Geometry check sheet. Reference: drawing and pictorial views, mm from the part's lowest x, y, z. Give positions to 0.01 mm unless a question says otherwise; leave off trailing zeros. Order: outer loops, then holes, each group sorted by start corner. A loop starts at its lowest first (then second) coordinate and runs counter-clockwise, first axis right, second up.
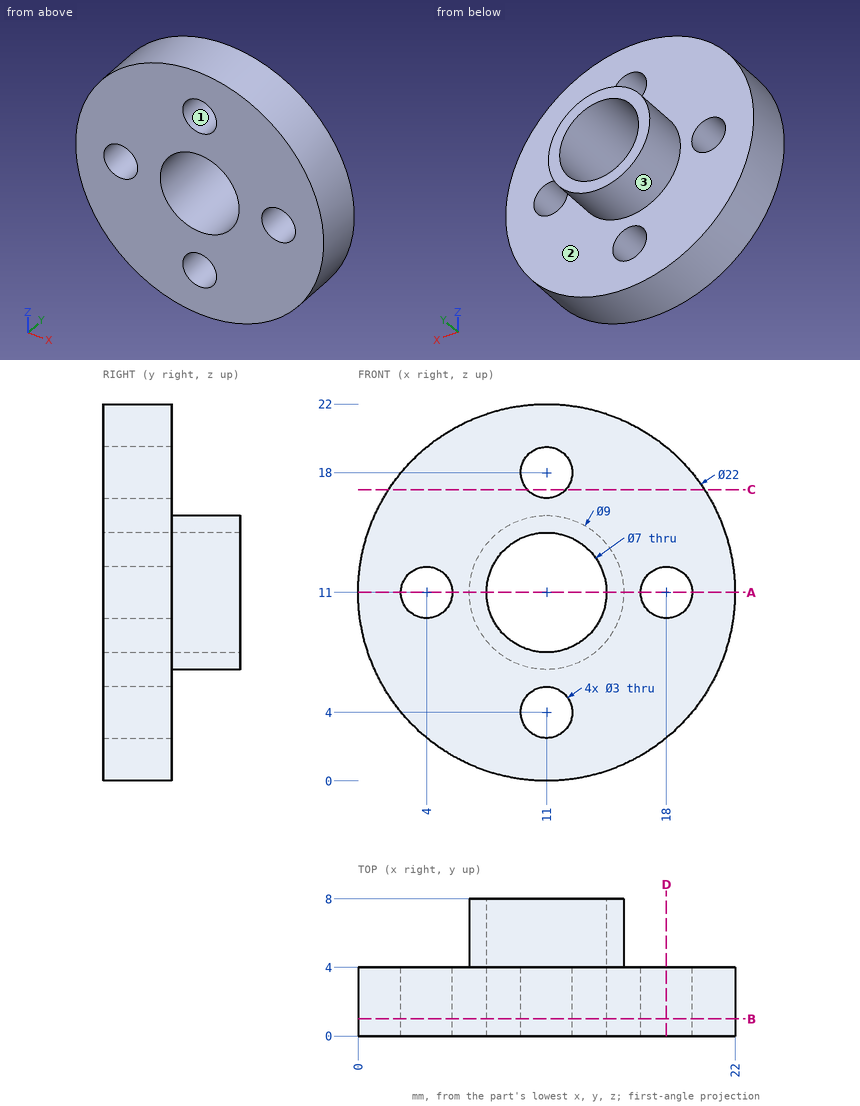
(1) Material ranges on L1, parallel to X at y = 0.9, z = 11; L2, parallel to Z at x = 10, y = 1.25; L3, parallel to Y at x = 5.75, z = 13.5, recorded low to high.
Response values:
L1: x = 0 to 2.5, 5.5 to 7.5, 14.5 to 16.5, 19.5 to 22
L2: z = 0.05 to 2.88, 5.12 to 7.65, 14.35 to 16.88, 19.12 to 21.95
L3: y = 0 to 4
(2) Cross-section at C-C on z = 17. Enter the section's corners in (x, y), then the cut area to 3 significant figures.
Response values:
outline: (1.78, 0) - (9.88, 0) - (9.88, 4) - (1.78, 4) - close; (12.12, 0) - (20.22, 0) - (20.22, 4) - (12.12, 4) - close
area: 64.8 mm2
(3) Cross-section at D-D on x = 18. Enter the section's corners in (y, z), then the cut area to 3 significant figures.
Response values:
outline: (0, 2.51) - (4, 2.51) - (4, 9.5) - (0, 9.5) - close; (0, 12.5) - (4, 12.5) - (4, 19.49) - (0, 19.49) - close
area: 55.9 mm2
(4) Release check for a two-part mould opening along Z. For the marked faces 1, 2 and 3 record: released by +Z, released by -Z, zero draft, split by the parting line, or undercut.
Response values:
face 1: undercut
face 2: zero draft
face 3: split by the parting line
(5) Cross-section at B-B on y = 1. Enter the section's corners in (x, z).
Response values:
outline: circle Ø22 at (11, 11); hole circle Ø3 at (4, 11); hole circle Ø7 at (11, 11); hole circle Ø3 at (11, 4); hole circle Ø3 at (11, 18); hole circle Ø3 at (18, 11)
(6) Cross-section at A-A on z = 11. Enter the section's corners in (x, y), then the cut area to 3 significant figures.
Response values:
outline: (0, 0) - (2.5, 0) - (2.5, 4) - (0, 4) - close; (5.5, 0) - (7.5, 0) - (7.5, 8) - (6.5, 8) - (6.5, 4) - (5.5, 4) - close; (14.5, 0) - (16.5, 0) - (16.5, 4) - (15.5, 4) - (15.5, 8) - (14.5, 8) - close; (19.5, 0) - (22, 0) - (22, 4) - (19.5, 4) - close
area: 44.0 mm2
(7) Gauge pin test, flat ends, axial feed: pin 1 Ø1 at (x, z) = (10, 12.5) entering from -Y; pin 2 Ø5 at (x, z) = (4, 16) entering from +Y; pin 3 Ø4 at (x, y) = (17, 3) entering from -Z. Record the tip position at first contact, or that the pin passes through.
Response values:
pin 1: passes through
pin 2: stops at y = 4
pin 3: stops at z = 0.75
